Autodesk Inventor part; units mm, degrees
ref_plane "YZ Plane" through (0, 0, 0) normal (1, 0, 0) x (0, 1, 0)
ref_plane "XZ Plane" through (0, 0, 0) normal (0, 1, 0) x (-1, 0, 0)
ref_plane "XY Plane" through (0, 0, 0) normal (0, 0, 1) x (1, 0, 0)
sketch "Boceto1" plane through (0, 0, 0) normal (1, 0, 0) x (0, 1, 0)
  line L0 (0, 0) -> (30, 0)
  line L1 (30, 0) -> (30, -20)
  line L2 (30, -20) -> (0, -20)
  line L3 (0, -20) -> (0, 0)
  line L4 (21, -10) -> (11, -10) construction
  line L5 (21, -7) -> (11, -7)
  line L6 (11, -13) -> (21, -13)
  arc A0 (21, -13) -> (21, -7) centre (21, -10) ccw
  arc A1 (11, -7) -> (11, -13) centre (11, -10) ccw
  point P0 (16, -10)
  point P1 (24, -10)
  point P2 (30, -10)
  point P3 (0, -10)
  point P4 (8, -10)
  dimension "d0" = 30
  dimension "d1" = 20
  dimension "d2" = 10
  dimension "d3" = 6
  dimension "d4" = 6
extrude "Extrusión1" add sketch "Boceto1" along normal blind 5
sketch "Boceto2" plane through (5, 0, 0) normal (1, 0, 0) x (0, 0, -1)
  line L0 (0, 0) -> (20, 0)
  line L1 (0, 0) -> (20, 0)
  line L2 (20, 0) -> (20, 5)
  line L3 (20, 5) -> (0, 5)
  line L4 (0, 5) -> (0, 0)
  dimension "d8" = 20
  dimension "d9" = 5
extrude "Extrusión2" add sketch "Boceto2" along normal blind 25
sketch "Boceto3" plane through (5, 5, 0) normal (0, 1, 0) x (1, 0, 0)
  line L0 (6, 10) -> (16, 10) construction
  line L1 (6, 7) -> (16, 7)
  line L2 (16, 13) -> (6, 13)
  arc A0 (6, 13) -> (6, 7) centre (6, 10) ccw
  arc A1 (16, 7) -> (16, 13) centre (16, 10) ccw
  line L3 (25, 20) -> (25, 0)
  line L4 (0, 0) -> (25, 0)
  point P0 (-5, 0)
  point P1 (11, 10)
  point P2 (25, 10)
  point P3 (19, 10)
  dimension "d12" = 10
  dimension "d13" = 6
  dimension "d14" = 6
  dimension "d15" = 10
extrude "Extrusión3" cut sketch "Boceto3" against normal blind 5
sketch "Boceto4" plane through (0, 0, 0) normal (0, 0, 1) x (1, 0, 0)
  line L0 (5, 30) -> (5, 5)
  line L1 (5, 5) -> (30, 5)
  line L2 (5, 5) -> (5, 28)
  line L3 (5, 30) -> (7, 30)
  line L4 (7, 30) -> (7, 28)
  line L5 (30, 5) -> (30, 7)
  line L6 (30, 7) -> (28, 7)
  line L7 (28, 7) -> (7, 28)
  point P0 (0, 0)
  point P1 (28, 5)
  dimension "d18" = 2
  dimension "d19" = 2
  dimension "d22" = 2
extrude "Extrusión4" add sketch "Boceto4" against normal blind 2
sketch "Boceto5" plane through (0, 0, -20) normal (0, 0, -1) x (-1, 0, 0)
  line L0 (-30, 0) -> (-30, 5)
  line L1 (-30, 0) -> (-30, 7)
  line L2 (-30, 5) -> (-30, 7)
  line L3 (-30, 7) -> (-28, 7)
  line L4 (-7, 30) -> (-7, 28)
  line L5 (-28, 7) -> (-7, 28)
  line L6 (-7, 28) -> (-7, 30)
  line L7 (-7, 30) -> (-5, 30)
  line L8 (-5, 30) -> (-5, 5)
  line L9 (-5, 5) -> (-30, 5)
  point P0 (0, 0)
  dimension "d23" = 2
extrude "Extrusión5" add sketch "Boceto5" against normal blind 5
sketch "Boceto6" plane through (0, 0, 0) normal (0, 0, 1) x (1, 0, 0)
  line L0 (28, 7) -> (7, 28)
  line L1 (7, 28) -> (7, 13)
  line L2 (7, 13) -> (13, 7)
  line L3 (13, 7) -> (28, 7)
  point P0 (0, 0)
  dimension "d26" = 45
  dimension "d27" = 15
extrude "Extrusión6" cut sketch "Boceto6" against normal blind 2
sketch "Boceto7" plane through (0, 0, -15) normal (0, 0, 1) x (1, 0, 0)
  line L0 (7, 28) -> (28, 7)
  line L1 (7, 28) -> (7, 7)
  line L2 (7, 7) -> (28, 7)
  line L3 (7, 7) -> (17.5, 17.5)
  line L4 (28, 7) -> (7, 28)
  point P0 (0, 0)
  point P1 (13.9645, 13.9645)
  point P2 (17.5, 17.5)
  dimension "d30" = 5
hole "Agujero1" at (13.9645, 13.9645, -15) direction (0, 0, -1) diameter 2 end through all
properties part number "Esquinero"
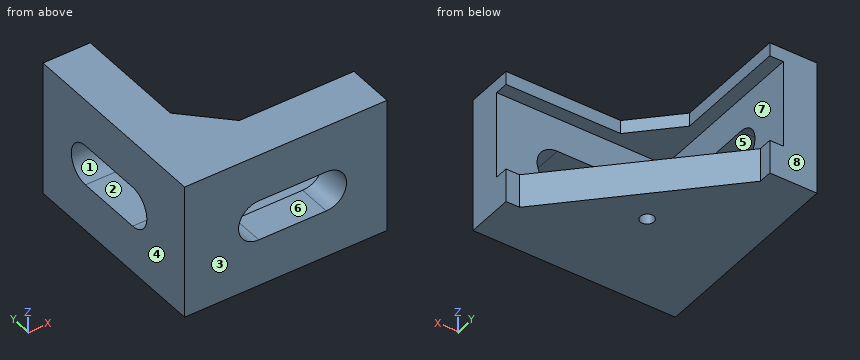
Read the model definition and answer for the solid it produces. Units are mm, in the model's axes. Face numbers are marked on the shaded views. A direction names the side the tool comes from. Round coordinates to 2 decimals unless told otherwise and drop trailing zeros. Loops run counter-clockwise (first coordinate to the right, second up) from the corner with the lowest first, then second, coordinate; pieces in that order, holes last. Notation, with made-up numbers: (82, 61.25) -> (93, 61.25) arc R15 ccw to (93, 72.25) -> close; hole circle Ø5 at (-2.75, 76). An arc over 180 degrees is marked (long way). One line per item, written item: value.
1) The mould has two halves that part along Y. Classify the marked faces 1, 2, 3 and 4: pulls with the +Y half, pulls with the -Y half, needs draft (parallel to the pull), parting line crosses it, or undercut.
Answer list:
face 1: undercut
face 2: undercut
face 3: pulls with the -Y half
face 4: needs draft
2) A cutting plane is placed at B-B (y = 12). Determine the outline of the cut face in (x, z), and give its area (3 significant figures).
Answer list:
outline: (0, -20) -> (23, -20) -> (23, -15) -> (5, -15) -> (5, -13) -> (0, -13) -> close; (0, -7) -> (5, -7) -> (5, -2) -> (8, -2) -> (8, 0) -> (0, 0) -> close
area: 166 mm²
3) A cutting plane is placed at A-A (z = -10). Determine the outline of the cut face in (x, y), and give its area (3 significant figures).
Answer list:
outline: (0, 0) -> (8, 0) -> (8, 5) -> (5, 5) -> (5, 8) -> (0, 8) -> close; (0, 24) -> (5, 24) -> (5, 30) -> (0, 30) -> close; (24, 0) -> (30, 0) -> (30, 5) -> (24, 5) -> close
area: 115 mm²
4) For the marked faces 5, 6, 7 and 8, determine the directions among +Z, -Z, +X, -X, +Y, -Y from which every point of the face is accessible in a straight line to the end or side of a thin tool.
Answer list:
face 5: +X, -X
face 6: +Y, -Y
face 7: +X, +Y
face 8: +Z, -Z, +X, -X, +Y
5) Flat-ended cylindrical pins translate along their axes: P1, Ø5, axis at y = 8.5, z = -12, coming from the +X side; P2, Ø1, axis at x = 16, z = -3.5, coming from the +Y side; P3, Ø2, axis at y = 19.5, z = -1, coming from the +X side. Find the tip coordinate at first contact, or state that the pin passes through.
Answer list:
P1: stops at x = 5
P2: stops at y = 5
P3: stops at x = 7
6) Consider L1, parallel to Z at x = 6.5, y = 21.5; L2, parallel to Y at x = 19, z = -14. Determine where each line is inside the solid, lowest interval first. Write a range as [from, to].
Answer list:
L1: z = [-20, -15], [-2, 0]
L2: y = [0, 5]
7) A cutting plane is placed at D-D (x = 13.5). Determine the outline of the cut face in (y, z), and give its area (3 significant figures).
Answer list:
outline: (0, -20) -> (13.08, -20) -> (13.08, -15) -> (5, -15) -> (5, -13) -> (0, -13) -> close; (0, -7) -> (5, -7) -> (5, -2) -> (7, -2) -> (7, 0) -> (0, 0) -> close; (14.85, -20) -> (21.5, -20) -> (21.5, -15) -> (14.85, -15) -> close
area: 148 mm²
8) A cutting plane is placed at C-C (x = 10). Determine the outline of the cut face in (y, z), and give its area (3 significant figures).
Answer list:
outline: (0, -20) -> (25, -20) -> (25, -15) -> (5, -15) -> (5, -12.83) -> (0, -12.83) -> close; (0, -7.17) -> (5, -7.17) -> (5, -2) -> (10, -2) -> (10, 0) -> (0, 0) -> close
area: 182 mm²
